Can you work these out from the model? Positions are in its coordinate system, mm. Face numbers are marked on the shaded views. A direction names the side the tool comes from. Give positions to 0.01 mm unless a question says otherwise; leave off trailing zeros. Order: outer loops, then holes, each group sorted by start corner. A loop starts at its lowest first (then second) coordinate and runs counter-clockwise, first axis right, second up. Notation, with made-up numbers: M 80,-2 L 94,-2 A18 cw 94,3 Z; hole C -7,27.5 d1. An arc over 180 degrees is marked long. Answer as a JSON object with one key per item and string values.
```python
from build123d import *

# Parameters (mm, degrees)
GENERAL_EXTRUDE_DEPTH       = 459.76
ROUNDING_R                  = 5
ROLLER_HOLDERS_DEPTH        = 461.873363952
SKETCH5_W                   = 5
SKETCH5_H                   = 919.52
GUARD_RAIL_DEPTH            = 100
GUARD_RAIL_SUPPORT_FILLET_R = 5


with BuildPart() as part:
    # Sketch2 → General extrude (new, symmetric)
    with BuildSketch(Plane.XY):
        Polygon((-12.5, 20), (-12.5, -20), (12.5, -20), (12.5, -15), (2.5, -15), (2.5, 20), align=None)
    extrude(amount=GENERAL_EXTRUDE_DEPTH, both=True)

    # Rounding
    rounding_edges = [part.edges().sort_by_distance(p)[0] for p in [
        (2.5, 20, 0),
        (2.5, -15, 0),
    ]]
    fillet(rounding_edges, radius=ROUNDING_R)

    # Sketch3 → Roller holders (cut, through all)
    with BuildSketch(Plane.ZY.offset(12.5)):
        Polygon((436.967180745, 3.89), (440.174361491, 9.445), (436.967180745, 15), (430.552819255, 15), (427.345638509, 9.445), (430.552819255, 3.89), align=None)
        Polygon((379.137180745, 3.89), (382.344361491, 9.445), (379.137180745, 15), (372.722819255, 15), (369.515638509, 9.445), (372.722819255, 3.89), align=None)
        Polygon((321.307180745, 3.89), (324.514361491, 9.445), (321.307180745, 15), (314.892819255, 15), (311.685638509, 9.445), (314.892819255, 3.89), align=None)
        Polygon((263.477180745, 3.89), (266.684361491, 9.445), (263.477180745, 15), (257.062819255, 15), (253.855638509, 9.445), (257.062819255, 3.89), align=None)
        Polygon((205.647180745, 3.89), (208.854361491, 9.445), (205.647180745, 15), (199.232819255, 15), (196.025638509, 9.445), (199.232819255, 3.89), align=None)
        Polygon((147.817180745, 3.89), (151.024361491, 9.445), (147.817180745, 15), (141.402819255, 15), (138.195638509, 9.445), (141.402819255, 3.89), align=None)
        Polygon((89.987180745, 3.89), (93.194361491, 9.445), (89.987180745, 15), (83.572819255, 15), (80.365638509, 9.445), (83.572819255, 3.89), align=None)
        Polygon((32.157180745, 3.89), (35.364361491, 9.445), (32.157180745, 15), (25.742819255, 15), (22.535638509, 9.445), (25.742819255, 3.89), align=None)
        Polygon((-25.672819255, 3.89), (-22.465638509, 9.445), (-25.672819255, 15), (-32.087180745, 15), (-35.294361491, 9.445), (-32.087180745, 3.89), align=None)
        Polygon((-83.502819255, 3.89), (-80.295638509, 9.445), (-83.502819255, 15), (-89.917180745, 15), (-93.124361491, 9.445), (-89.917180745, 3.89), align=None)
        Polygon((-141.332819255, 3.89), (-138.125638509, 9.445), (-141.332819255, 15), (-147.747180745, 15), (-150.954361491, 9.445), (-147.747180745, 3.89), align=None)
        Polygon((-199.162819255, 3.89), (-195.955638509, 9.445), (-199.162819255, 15), (-205.577180745, 15), (-208.784361491, 9.445), (-205.577180745, 3.89), align=None)
        Polygon((-256.992819255, 3.89), (-253.785638509, 9.445), (-256.992819255, 15), (-263.407180745, 15), (-266.614361491, 9.445), (-263.407180745, 3.89), align=None)
        Polygon((-314.822819255, 3.89), (-311.615638509, 9.445), (-314.822819255, 15), (-321.237180745, 15), (-324.444361491, 9.445), (-321.237180745, 3.89), align=None)
        Polygon((-372.652819255, 3.89), (-369.445638509, 9.445), (-372.652819255, 15), (-379.067180745, 15), (-382.274361491, 9.445), (-379.067180745, 3.89), align=None)
        Polygon((-430.482819255, 3.89), (-427.275638509, 9.445), (-430.482819255, 15), (-436.897180745, 15), (-440.104361491, 9.445), (-436.897180745, 3.89), align=None)
    extrude(amount=-ROLLER_HOLDERS_DEPTH, mode=Mode.SUBTRACT)

    # Sketch5 → Guard rail (add)
    with BuildSketch(Plane(origin=(0, 20, 0), x_dir=(1, 0, 0), z_dir=(0, 1, 0))):
        with Locations((-10, 0)):
            Rectangle(SKETCH5_W, SKETCH5_H)
    extrude(amount=GUARD_RAIL_DEPTH)

    # Guard rail support fillet
    guard_rail_support_fillet_edges = [part.edges().sort_by_distance(p)[0] for p in [
        (-7.5, 20, 0),
    ]]
    fillet(guard_rail_support_fillet_edges, radius=GUARD_RAIL_SUPPORT_FILLET_R - 0.0001)  # a hair under: the kernel refuses the full size


solid = part.part
```
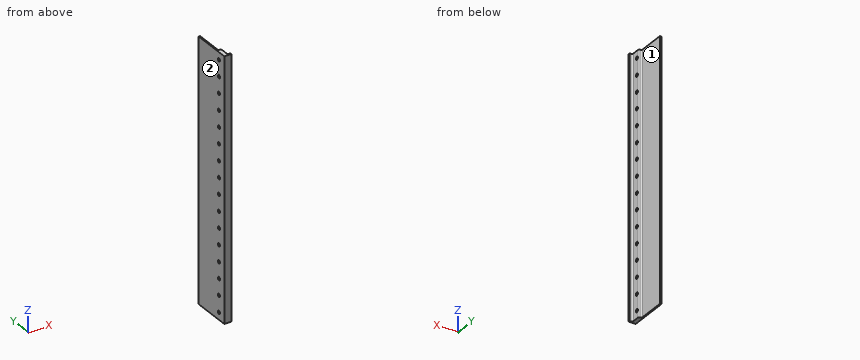
1) For the marked faces 1 and 2, which set-ups out of +Z, -Z, +X, -X, +Y, -Y let a thin tool reach every point of the face, with its end or its side?
Results found:
{"face 1": "+Z, -Z, +X, +Y", "face 2": "+Z, -Z, -X, +Y, -Y"}
2) I need wall thicknesses on L1, parallel to Y at x = -3.25, z = -261; L2, parallel to X at y = 27, z = 228; L3, parallel to Y at x = -0.5, z = 139. Which ranges of each line are inside material? Lowest first, please.
Results found:
{"L1": "y = -20 to 3.89, 15 to 20.06", "L2": "x = -12.5 to -7.5", "L3": "y = -20 to 8.05, 10.84 to 19.58"}
3) I want a section at B-B on y = 102. Write out the boundary of the cut face in (x, z), and give its area (3 significant figures).
Results found:
{"outline": "M -12.5,-459.76 L -7.5,-459.76 L -7.5,459.76 L -12.5,459.76 Z", "area": "4,600 mm²"}
4) I'm going to push flat-ended pins straight in: pin 1 Ø3 at (x, z) = (-4.5, 377) entering from +Y; pin 2 Ø7 at (x, z) = (-2, -144) entering from +Y; pin 3 Ø1 at (x, z) = (5.5, 164.5) entering from +Y. Where does each tip first touch, or does it pass through?
Results found:
{"pin 1": "stops at y = 21.43", "pin 2": "stops at y = 21", "pin 3": "stops at y = -14.33"}
